Input: dimensioned drawing with shaded views. Units: mm. Origin: part minimum x, y, z. A direction names the side the tool comes from. Round coordinates to 2 decimals unless told otherwise and drop trailing zeros. Order: outer loops, then holes, each group sorted by start corner. A loop starts at its lowest first (then second) coordinate and runs counter-clockwise, first axis right, second up. Notation, with made-up numbers: (37, 42.5) - (92, 42.5) arc R27 cw to (92, 70.5) - close; hole circle Ø5 at (69.25, -37.75). An arc over 180 degrees is marked (long way). Return JSON: item names as keys, results as strings. Group by question number.
1) Section C-C, the plane y = 171.5. Return loops of the section in (x, z), plus the area to 3 significant figures.
2) Mould query, pull axis Y, two halves, no side actions, for the marked faces 1, 2, 3 and 4. Classes: pulls with the +Y half, pulls with the -Y half, needs draft (parallel to the pull), parting line crosses it, or undercut.
3) Section A-A, the plane z = 15.5. Return loops of the section in (x, y).
4) Contact query for flat-ended pins moving along their axis: P1, Ø10, axis at y = 98.5, z = 7.5, coming from the -X side; P2, Ø8, axis at x = 195, y = 64.5, coming from the +Z side. Output: stop coordinate, or through.
5) Access query for the marked faces 5 and 6. Directions: +Z, -Z, +X, -X, +Y, -Y. A direction counts if a zero-diameter tool reaches every point of the face in a straight line with its end or side. Return the directions, or none.
6) Section D-D, the plane x = 75. Return loops of the section in (y, z), plus the area to 3 significant figures.
7) Section B-B, the plane x = 180. Return loops of the section in (y, z), plus the area to 3 significant figures.
8) Ray query, line 1 (Z direction, x = 120.5, y = 145); line 2 (Y direction, x = 155, z = 12.5); line 3 (Z direction, x = 97, y = 131). Return the intervals inside material, ascending. Write a range as from..to.
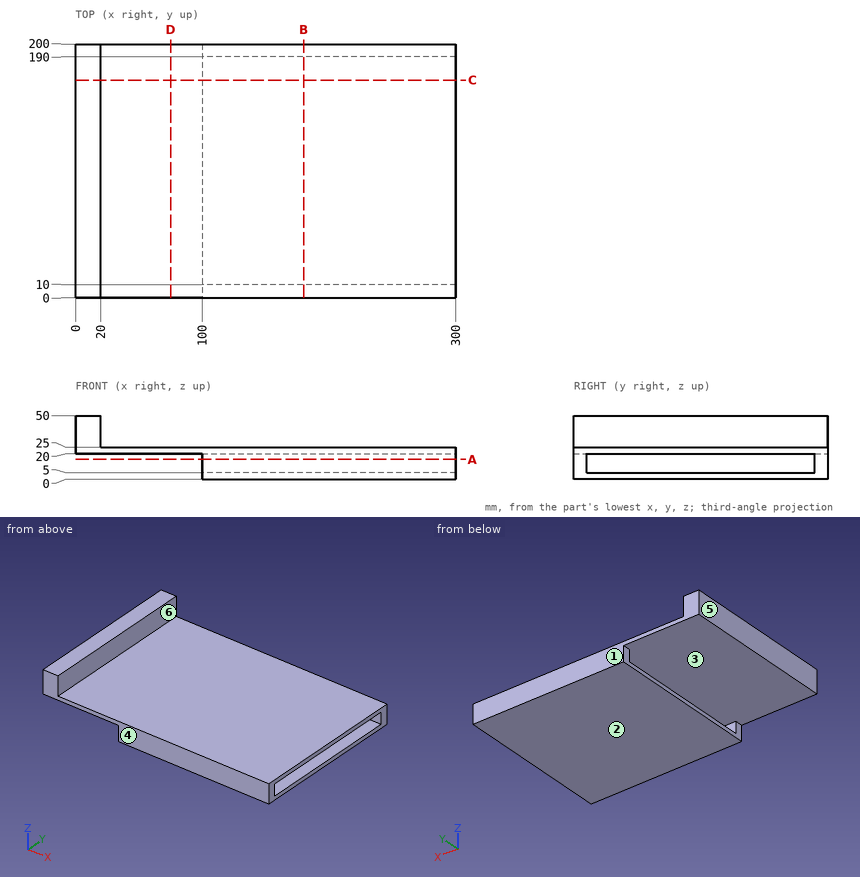
Geometry check:
{
 "1": {"outline": "(0, 20) - (300, 20) - (300, 25) - (20, 25) - (20, 50) - (0, 50) - close; (100, 0) - (300, 0) - (300, 5) - (100, 5) - close", "area": "3,000 mm2"},
 "2": {"face 1": "pulls with the +Y half", "face 2": "needs draft", "face 3": "undercut", "face 4": "pulls with the -Y half"},
 "3": {"outline": "(100, 0) - (300, 0) - (300, 10) - (100, 10) - close; (100, 190) - (300, 190) - (300, 200) - (100, 200) - close"},
 "4": {"P1": "x = 100", "P2": "z = 25"},
 "5": {"face 5": "+Z, -Z, -X, +Y, -Y", "face 6": "+Z, +X, +Y, -Y"},
 "6": {"outline": "(0, 20) - (200, 20) - (200, 25) - (0, 25) - close", "area": "1,000 mm2"},
 "7": {"outline": "(0, 0) - (200, 0) - (200, 25) - (0, 25) - close; hole (10, 5) - (190, 5) - (190, 20) - (10, 20) - close", "area": "2,300 mm2"},
 "8": {"line 1": "0..5, 20..25", "line 2": "0..10, 190..200", "line 3": "20..25"}
}
